Check sheet for the modelled part. Datum: model origin and axes. Units: mm. Face numbers are marked on the shaded views. A direction names the side the tool comes from. Round coordinates to 2 decimals unless told otherwise and drop trailing zeros. Order: outer loops, then holes, each group sorted by start corner. A loop starts at its lowest first (then second) coordinate and runs counter-clockwise, first axis right, second up. Notation, with made-up numbers: M -16.75,53.25 L 5.25,53.25 A21 ccw 5.25,71.25 Z; hole C -34,86.5 d5. An arc over 180 degrees is marked long. One line per item, written item: value. Start each with the question number.
(1) Cross-section at A-A, the plane y = 197. Enter the section's corners in (x, z) (3 decimals), and give its area (3 significant figures).
(2) Thickness scan on L1, parallel to X at y = 355, z = -1.7 (3 decimals); L2, parallel to X at y = 273.5, z = -19 (3 decimals); L3, parallel to Z at x = 6.5, y = 421.5 (3 decimals). Record the ranges inside material, lowest first.
(3) Depth check by flat-ended pin: pin 1 Ø5 at (x, y) = (23.81, 7.94) entering from +Z; pin 2 Ø3 at (x, y) = (14.29, 319.9) entering from +Z; pin 3 Ø8 at (x, y) = (8.5, 257.5) entering from -Z (3 decimals); pin 4 Ø6 at (y, z) = (358, -15.5) entering from +X (3 decimals). Enter the tip coordinate at first touch or a pass-through.
(4) Access from +Z, -Z, +X, -X, +Y, -Y to the whole of each face (thin tool, end or side, straight path). Record for the marked faces 1 and 2.
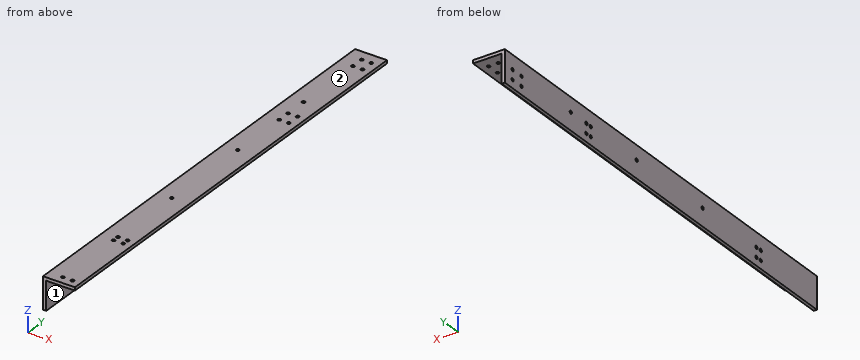
from build123d import *

# Parameters (mm, degrees)
BOSS_EXTRUDE1_DEPTH              = 450
LEFTSIDEHOLES_SKETCH3_R          = 1.5875
LEFTSIDEHOLES_CUT_EXTRUDE1_DEPTH = 3.175
BACKSIDEHOLES_SKETCH4_R          = 1.5875
BACKSIDEHOLES_CUT_EXTRUDE2_DEPTH = 3.175


with BuildPart() as part:
    # Sketch2 → Boss-Extrude1 (new body)
    with BuildSketch(Plane(origin=(0, 0, 0), x_dir=(1, 0, 0), z_dir=(0, 1, 0))):
        Polygon((0, 31.75), (3.175, 31.75), (3.175, 3.175), (31.75, 3.175), (31.75, 0), (0, 0), align=None)
    extrude(amount=BOSS_EXTRUDE1_DEPTH)

    # LeftSideHoles-Sketch3 → LeftSideHoles-Cut-Extrude1 (cut)
    with BuildSketch(Plane.XY):
        with Locations((14.2875, 81.1125)):
            Circle(LEFTSIDEHOLES_SKETCH3_R)
        with Locations((23.8125, 81.1125)):
            Circle(LEFTSIDEHOLES_SKETCH3_R)
        with Locations((14.2875, 87.4625)):
            Circle(LEFTSIDEHOLES_SKETCH3_R)
        with Locations((23.8125, 87.4625)):
            Circle(LEFTSIDEHOLES_SKETCH3_R)
        with Locations((14.2875, 438.8875)):
            Circle(LEFTSIDEHOLES_SKETCH3_R)
        with Locations((14.2875, 426.1875)):
            Circle(LEFTSIDEHOLES_SKETCH3_R)
        with Locations((23.8125, 438.8875)):
            Circle(LEFTSIDEHOLES_SKETCH3_R)
        with Locations((23.8125, 426.1875)):
            Circle(LEFTSIDEHOLES_SKETCH3_R)
        with Locations((14.2875, 332.602644)):
            Circle(LEFTSIDEHOLES_SKETCH3_R)
        with Locations((23.8125, 332.602644)):
            Circle(LEFTSIDEHOLES_SKETCH3_R)
        with Locations((14.2875, 319.902644)):
            Circle(LEFTSIDEHOLES_SKETCH3_R)
        with Locations((23.8125, 319.902644)):
            Circle(LEFTSIDEHOLES_SKETCH3_R)
        with Locations((14.2875, 7.9375)):
            Circle(LEFTSIDEHOLES_SKETCH3_R)
        with Locations((23.8125, 7.9375)):
            Circle(LEFTSIDEHOLES_SKETCH3_R)
        with Locations((14.2875, 165)):
            Circle(LEFTSIDEHOLES_SKETCH3_R)
        with Locations((14.2875, 260)):
            Circle(LEFTSIDEHOLES_SKETCH3_R)
        with Locations((14.2875, 355)):
            Circle(LEFTSIDEHOLES_SKETCH3_R)
    extrude(amount=-LEFTSIDEHOLES_CUT_EXTRUDE1_DEPTH, mode=Mode.SUBTRACT)

    # BackSideHoles-Sketch4 → BackSideHoles-Cut-Extrude2 (cut)
    with BuildSketch(Plane.ZY):
        with Locations((-23.8125, 81.1125)):
            Circle(BACKSIDEHOLES_SKETCH4_R)
        with Locations((-14.2875, 81.1125)):
            Circle(BACKSIDEHOLES_SKETCH4_R)
        with Locations((-23.8125, 87.4625)):
            Circle(BACKSIDEHOLES_SKETCH4_R)
        with Locations((-14.2875, 87.4625)):
            Circle(BACKSIDEHOLES_SKETCH4_R)
        with Locations((-23.8125, 438.8875)):
            Circle(BACKSIDEHOLES_SKETCH4_R)
        with Locations((-14.2875, 438.8875)):
            Circle(BACKSIDEHOLES_SKETCH4_R)
        with Locations((-23.8125, 426.1875)):
            Circle(BACKSIDEHOLES_SKETCH4_R)
        with Locations((-14.2875, 426.1875)):
            Circle(BACKSIDEHOLES_SKETCH4_R)
        with Locations((-23.8125, 332.602644)):
            Circle(BACKSIDEHOLES_SKETCH4_R)
        with Locations((-14.2875, 332.602644)):
            Circle(BACKSIDEHOLES_SKETCH4_R)
        with Locations((-23.8125, 326.252644)):
            Circle(BACKSIDEHOLES_SKETCH4_R)
        with Locations((-14.2875, 326.252644)):
            Circle(BACKSIDEHOLES_SKETCH4_R)
        with Locations((-14.2875, 165)):
            Circle(BACKSIDEHOLES_SKETCH4_R)
        with Locations((-14.2875, 260)):
            Circle(BACKSIDEHOLES_SKETCH4_R)
        with Locations((-14.2875, 355)):
            Circle(BACKSIDEHOLES_SKETCH4_R)
    extrude(amount=-BACKSIDEHOLES_CUT_EXTRUDE2_DEPTH, mode=Mode.SUBTRACT)


solid = part.part
Values found:
1. outline: M 0,-31.75 L 3.175,-31.75 L 3.175,-3.175 L 31.75,-3.175 L 31.75,0 L 0,0 Z
1. area: 192 mm^2
2. L1: 0 to 12.7, 15.875 to 31.75
2. L2: 0 to 3.175
2. L3: -3.175 to 0
3. pin 1: z = 0
3. pin 2: through
3. pin 3: z = -3.175
3. pin 4: x = 3.175
4. face 1: -Z, +X, +Y, -Y
4. face 2: +Z, +X, -X, +Y, -Y
